from build123d import *

# Parameters (mm, degrees)
SKETCH1_R                = 28.575
SKETCH1_R_2              = 15.875
BOSS_EXTRUDE1_DEPTH      = 6.35
BOSS_EXTRUDE2_DEPTH      = 6.35
F_0_257_DIAMETER_HOLE1_D = 6.5278
CIRPATTERN1_COUNT        = 4
CUT_EXTRUDE1_DEPTH       = 7.35
FILLET1_R                = 5.08
SKETCH6_R                = 2.15265
CUT_EXTRUDE2_DEPTH       = 7.35


with BuildPart() as part:
    # Sketch1 → Boss-Extrude1 (new body)
    with BuildSketch(Plane(origin=(0, 0, 0), x_dir=(1, 0, 0), z_dir=(0, 1, 0))):
        Circle(SKETCH1_R)
        Circle(SKETCH1_R_2, mode=Mode.SUBTRACT)
    extrude(amount=BOSS_EXTRUDE1_DEPTH)

    # Sketch2 → Boss-Extrude2 (add)
    with BuildSketch(Plane(origin=(0, 6.35, 0), x_dir=(1, 0, 0), z_dir=(0, 1, 0))):
        with BuildLine():
            Line((73.025, -7.9375), (25.4, -7.9375))
            Line((25.4, -7.9375), (25.4, 7.9375))
            Line((25.4, 7.9375), (73.025, 7.9375))
            ThreePointArc((73.025, 7.9375), (77.515128061, 6.077628061), (79.375, 1.5875))
            Line((79.375, 1.5875), (79.375, -1.5875))
            ThreePointArc((79.375, -1.5875), (77.515128061, -6.077628061), (73.025, -7.9375))
        make_face()
        with BuildLine():
            Line((58.870802517, -3.175), (33.470802517, -3.175))
            ThreePointArc((33.470802517, -3.175), (30.295802517, 0), (33.470802517, 3.175))
            Line((33.470802517, 3.175), (58.870802517, 3.175))
            ThreePointArc((58.870802517, 3.175), (62.045802517, 0), (58.870802517, -3.175))
        make_face(mode=Mode.SUBTRACT)
    boss_extrude2 = extrude(amount=-BOSS_EXTRUDE2_DEPTH)

    # F (0.257) Diameter Hole1 (through all)
    with Locations(Plane(origin=(0, 6.35, 0), x_dir=(1, 0, 0), z_dir=(0, 1, 0))):
        with Locations((69.85, 0)):
            f_0_257_diameter_hole1 = Hole(F_0_257_DIAMETER_HOLE1_D / 2)

    # CirPattern1: Boss-Extrude2, F (0.257) Diameter Hole1 ×4 about axis
    cirpattern1_axis = Axis((0, 0, 0), (0, 1, 0))
    for i in range(1, CIRPATTERN1_COUNT):
        add(boss_extrude2.rotate(cirpattern1_axis, i * 360 / CIRPATTERN1_COUNT))
        add(f_0_257_diameter_hole1.rotate(cirpattern1_axis, i * 360 / CIRPATTERN1_COUNT), mode=Mode.SUBTRACT)

    # Sketch5 → Cut-Extrude1 (cut, through all)
    with BuildSketch(Plane(origin=(0, 6.35, 0), x_dir=(1, 0, 0), z_dir=(0, 1, 0))):
        Polygon((-7.9375, 19.830441139), (-7.9375, 27.450441139), (-7.9375, 52.536571615), (-88.152777481, 52.536571615), (-88.152777481, -52.536571615), (-7.9375, -52.536571615), (-7.9375, -27.450441139), (-7.9375, -19.830441139), (3.4925, -15.486060466), (3.4925, 15.486060466), align=None)
    extrude(amount=-CUT_EXTRUDE1_DEPTH, mode=Mode.SUBTRACT)

    # Fillet1
    fillet1_edges = [part.edges().sort_by_distance(p)[0] for p in [
        (-7.9375, 3.175, 19.830441139),
        (-7.9375, 3.175, -19.830441139),
    ]]
    fillet(fillet1_edges, radius=FILLET1_R)

    # Sketch6 → Cut-Extrude2 (cut, through all)
    with BuildSketch(Plane(origin=(0, 6.35, 0), x_dir=(1, 0, 0), z_dir=(0, 1, 0))):
        with Locations((-1.5875, 22.86)):
            Circle(SKETCH6_R)
        with Locations((-1.5875, -22.86)):
            Circle(SKETCH6_R)
    extrude(amount=-CUT_EXTRUDE2_DEPTH, mode=Mode.SUBTRACT)


solid = part.part
Here's how the part is built. I have some questions about the finished solid (model axes, mm). A direction names the side the tool comes from. Round coordinates to 2 decimals unless told otherwise and drop trailing zeros. Loops run counter-clockwise (first coordinate to the right, second up) from the corner with the lowest first, then second, coordinate; pieces in that order, holes last. Notation, with made-up numbers: (60, -39) - (91, -39) arc R22 cw to (91, -2) - close; hole circle Ø2 at (-17, -24). An arc over 180 degrees is marked (long way). One line per question, with ' | ' between items. Start each with the question number.
Q1. I want a section at C-C (z = 0). Write out the boundary of the cut face in (x, y) (3 decimals), then the cut area to 3 significant figures.
Q2. Please list where these lines run through material, in increasing order: line 1 (X direction, y = 1.5, z = 43.5) (1 decimal); line 2 (X direction, y = 1.5, z = 69.85). Write a range as [from, to].
Q3. I want a section at B-B (x = 69.85). Write out the boundary of the cut face in (y, z), then the cut area to 3 significant figures.
Q4. I want a section at D-D (y = 2.25). State how many separate pieces and enclosed holes the cut face has, then the cut area to 3 significant figures.
Q5. For faces 1 (the flat face through (46, 3, 3.175)), 2 (the flat face through (0, 3, -79.375)), 3 (the flat face through (-0.528, 3.219, -17.014)), which set-ups out of +Z, -Z, +X, -X, +Y, -Y let a thin tool reach every point of the face, with its end or its side?
Q6. We'd pull the mould along Z, two halves only. Please class faces 4 (the cylindrical face through (0.07, 3.219, -30.297)), 5 (the flat face through (46, 3, -3.175)), 6 (the flat face through (7.937, 3, 50)), 7 (the cylindrical face through (6.127, 3.219, 77.465)): +Z half, -Z half, draft (parallel to the pull), parting line (faces both ways), or undercut.
Q7. Will these pins go through, and if not, where does the flat tip stop? pin 1 (6 mm diameter, centred on x = 69.85, z = 0, fed in from +Y); pin 2 (3 mm diameter, centred on y = 3, z = -52, fed in from +X); pin 3 (1.5 mm diameter, centred on x = 48.5, y = 3.5, fed in from +Z); pin 4 (1.9 mm diameter, centred on x = 41.5, y = 2.5, fed in from -Z).
Response values:
1) outline: (15.875, 0) - (30.296, 0) - (30.296, 6.35) - (15.875, 6.35) - close; (62.046, 0) - (66.586, 0) - (66.586, 6.35) - (62.046, 6.35) - close; (73.114, 0) - (79.375, 0) - (79.375, 6.35) - (73.114, 6.35) - close | area: 160 mm²
2) line 1: x = [-7.9, -3.2], [3.2, 7.9] | line 2: x = [-7.94, -3.26], [3.26, 7.94]
3) outline: (0, -7.94) - (6.35, -7.94) - (6.35, -3.26) - (0, -3.26) - close; (0, 3.26) - (6.35, 3.26) - (6.35, 7.94) - (0, 7.94) - close | area: 59.4 mm²
4) separate pieces: 1 | enclosed holes: 8 | area: 2,710 mm²
5) face 1: +Y, -Y | face 2: -Z, +X, -X, +Y, -Y | face 3: -X, +Y, -Y
6) face 4: undercut | face 5: undercut | face 6: draft | face 7: +Z half
7) pin 1: passes through | pin 2: stops at x = 7.94 | pin 3: stops at z = 7.94 | pin 4: stops at z = -7.94
